```python
from build123d import *

# Parameters (mm, degrees)
SKETCH1_W           = 42
SKETCH1_H           = 90
SKETCH1_R           = 1.32
BOSS_EXTRUDE1_DEPTH = 6
SKETCH2_R           = 3.25
CUT_EXTRUDE1_DEPTH  = 5


with BuildPart() as part:
    # Sketch1 → Boss-Extrude1 (new body)
    with BuildSketch(Plane.XY):
        with Locations((0, -24.125)):
            Rectangle(SKETCH1_W, SKETCH1_H)
        with Locations((0, -15.875)):
            Circle(SKETCH1_R, mode=Mode.SUBTRACT)
        with Locations((-15.875, 0)):
            Circle(SKETCH1_R, mode=Mode.SUBTRACT)
        with Locations((0, 15.875)):
            Circle(SKETCH1_R, mode=Mode.SUBTRACT)
        with Locations((-9.53, -61.35)):
            Circle(SKETCH1_R, mode=Mode.SUBTRACT)
        with Locations((0, -61.35)):
            Circle(SKETCH1_R, mode=Mode.SUBTRACT)
        with Locations((9.53, -61.35)):
            Circle(SKETCH1_R, mode=Mode.SUBTRACT)
        with Locations((15.875, 0)):
            Circle(SKETCH1_R, mode=Mode.SUBTRACT)
    extrude(amount=BOSS_EXTRUDE1_DEPTH)

    # Sketch2 → Cut-Extrude1 (cut)
    with BuildSketch(Plane(origin=(0, 0, 0), x_dir=(-1, 0, 0), z_dir=(0, 0, -1))):
        with Locations((-15.875, 0)):
            Circle(SKETCH2_R)
        with Locations((0, 15.875)):
            Circle(SKETCH2_R)
        with Locations((15.875, 0)):
            Circle(SKETCH2_R)
        with Locations((0, -15.875)):
            Circle(SKETCH2_R)
    extrude(amount=-CUT_EXTRUDE1_DEPTH, mode=Mode.SUBTRACT)


solid = part.part
```
Here's how the part is built. I have some questions about the finished solid (model axes, mm). A direction names the side the tool comes from. Round coordinates to 2 decimals unless told otherwise and drop trailing zeros. Loops run counter-clockwise (first coordinate to the right, second up) from the corner with the lowest first, then second, coordinate; pieces in that order, holes last. Notation, with made-up numbers: (-24, -25) -> (12, -25) arc R20 cw to (12, -16) -> close; hole circle Ø9 at (-4, -24). An arc over 180 degrees is marked (long way). Answer as CSV lines item,"result".
1. Which directions (+Z, -Z, +X, -X, +Y, -Y) give clear straight access to the entire face, cutting with the end or side of a thin tool? Please do faces 1 (the face through (14, 0, 5)), 2 (the face through (-10.85, -61.29, 2.96)).
Final values:
face 1,"-Z"
face 2,"+Z, -Z"
2. If we section it at A-A on x = 9.53: Please give me the cut outline in (y, z) (3 decimals), plus the area to 3 significant figures.
Final values:
outline,"(-69.125, 0) -> (-62.67, 0) -> (-62.67, 6) -> (-69.125, 6) -> close; (-60.03, 0) -> (20.875, 0) -> (20.875, 6) -> (-60.03, 6) -> close"
area,"524 mm^2"
3. If we section it at D-D on x = 0: Please give me the cut outline in (y, z) (3 decimals), plus the area to 3 significant figures.
Final values:
outline,"(-69.125, 0) -> (-62.67, 0) -> (-62.67, 6) -> (-69.125, 6) -> close; (-60.03, 0) -> (-19.125, 0) -> (-19.125, 5) -> (-17.195, 5) -> (-17.195, 6) -> (-60.03, 6) -> close; (-14.555, 5) -> (-12.625, 5) -> (-12.625, 0) -> (12.625, 0) -> (12.625, 5) -> (14.555, 5) -> (14.555, 6) -> (-14.555, 6) -> close; (17.195, 5) -> (19.125, 5) -> (19.125, 0) -> (20.875, 0) -> (20.875, 6) -> (17.195, 6) -> close"
area,"454 mm^2"
4. If we section it at B-B on y = 0: Please give me the cut outline in (x, z) (3 decimals).
Final values:
outline,"(-21, 0) -> (-19.125, 0) -> (-19.125, 5) -> (-17.195, 5) -> (-17.195, 6) -> (-21, 6) -> close; (-14.555, 5) -> (-12.625, 5) -> (-12.625, 0) -> (12.625, 0) -> (12.625, 5) -> (14.555, 5) -> (14.555, 6) -> (-14.555, 6) -> close; (17.195, 5) -> (19.125, 5) -> (19.125, 0) -> (21, 0) -> (21, 6) -> (17.195, 6) -> close"
5. Thinking about a two-plate mould opening in X: for faces 3 (the face through (-21, -25, 3)), 4 (the face through (-12.63, 0.14, 2.46)), 5 (the face through (0, -23, 0)), 6 (the face through (0.61, -62.52, 2.96)), which applies, released by +X, released by -X, zero draft, split by the parting line, or undercut?
Final values:
face 3,"released by -X"
face 4,"undercut"
face 5,"zero draft"
face 6,"undercut"
6. If I drill on L1, parallel to Y at x = 0, z = 1.35 (3 decimals); L2, parallel to X at y = 0, z = 5.25 (3 decimals); L3, parallel to X at y = -2, z = 1.35, over which ranges is the centre line in solid material (lowest first)?
Final values:
L1,"y = -69.125 to -62.67, -60.03 to -19.125, -12.625 to 12.625, 19.125 to 20.875"
L2,"x = -21 to -17.195, -14.555 to 14.555, 17.195 to 21"
L3,"x = -21 to -18.44, -13.31 to 13.31, 18.44 to 21"
7. For pin 1 (2 mm diameter, centred on x = 0, y = -15.875, fed in from -Z); pin 2 (2 mm diameter, centred on x = 0, y = 17, fed in from -Z), each with a flat end and sliding along its axis, tell me the tip position at first contact or that it passes through.
Final values:
pin 1,"passes through"
pin 2,"stops at z = 5"
8. If we section it at C-C on z = 4.2: Please give me the cut outline in (x, y) (3 decimals), plus the area to 3 significant figures.
Final values:
outline,"(-21, -69.125) -> (21, -69.125) -> (21, 20.875) -> (-21, 20.875) -> close; hole circle Ø6.5 at (-15.875, 0); hole circle Ø2.64 at (-9.53, -61.35); hole circle Ø6.5 at (0, -15.875); hole circle Ø6.5 at (0, 15.875); hole circle Ø2.64 at (0, -61.35); hole circle Ø2.64 at (9.53, -61.35); hole circle Ø6.5 at (15.875, 0)"
area,"3,630 mm^2"
